Input: part model. Units: mm. Frame: model coordinates. A direction names the side the tool comes from. Coordinates: 2 decimals unless noted, no trailing zeros. Loops run counter-clockwise (first coordinate to the right, second up) from the corner with the lowest first, then second, coordinate; pieces in that order, holes last. Notation, with made-up numbers: M -8,-15.5 L 29,-15.5 A9 cw 29,-2.5 Z; hole C 21.25,-36.5 d11. An arc over 180 degrees is marked long. Use a Markdown table: item, result. Add a question column.
1. Section C-C on x = -12.5. Output: boundary loops of the cut face in (y, z), then the cut area to 3 significant figures.
2. Set-up query: faces 5 (the flat face through (0, -37, 1)), 6 (the cylindrical face through (-45.6, 35.5, 5)), 7 (the cylindrical face through (37.042, -47.174, 3.451)). Return all of +Z, -Z, +X, -X, +Y, -Y with unobstructed straight access to the full face (end or side cutting, diameter ignored); none if empty.
3. Line query: L1, parallel to Y at x = -10, z = 2; L2, parallel to X at y = -26.5, z = 5; L3, parallel to Y at x = 9, z = 6.5. Output: solid intervals per line, ascending. Write a range as [from, to].
4. Section B-B on z = 5.75. Output: boundary loops of the cut face in (x, y), then the cut area to 3 significant figures.
5. Section D-D on x = 19.5. Output: boundary loops of the cut face in (y, z).
6. Section A-A on y = -4. Output: boundary loops of the cut face in (x, z).
7. Pin query (flat end, axial travel): pin 1 (6 mm diameter, centred on x = 27, y = -1, fed in from +Z). Return the tip coordinate at first contact, or that it passes through.
8. Draft query along Y for faces 1 (the cylindrical face through (-41.951, 31.975, 1.521)), 2 (the cylindrical face through (-42.76, 21.16, 1.48)), 3 (the flat face through (14, -4, 0)), 4 (the cylindrical face through (-47.029, -47.096, 3.451)). Return one class per face: +Y half, -Y half, draft (parallel to the pull), parting line (faces both ways), or undercut.
```python
from build123d import *

# Parameters (mm, degrees)
F1_DEPTH = 3
F2_R     = 5
F3_R     = 5
F5_DEPTH = 4


with BuildPart() as f1:
    # F0 (on Top) → F1 (new body)
    with BuildSketch(Plane.XY):
        with BuildLine():
            Line((33.545249, 38.400311), (-43.454751, 38.400311))
            ThreePointArc((-43.454751, 38.400311), (-46.990285, 36.935845), (-48.454751, 33.400311))
            Line((-48.454751, 33.400311), (-48.454751, -43.599689))
            ThreePointArc((-48.454751, -43.599689), (-46.990285, -47.135222), (-43.454751, -48.599689))
            Line((-43.454751, -48.599689), (33.545249, -48.599689))
            ThreePointArc((33.545249, -48.599689), (37.080783, -47.135222), (38.545249, -43.599689))
            Line((38.545249, -43.599689), (38.545249, 33.400311))
            ThreePointArc((38.545249, 33.400311), (37.080783, 36.935845), (33.545249, 38.400311))
        make_face()
        with BuildLine():
            Line((-43.454751, 23.699071), (-43.454751, 33.400311))
            Line((-43.454751, 33.400311), (-2.236148, 33.400311))
            Line((-2.236148, 33.400311), (0, 33.400311))
            Line((0, 33.400311), (7.406416, 33.400311))
            ThreePointArc((7.406416, 33.400311), (8.481207, 33.201173), (9.41331, 32.630194))
            Line((9.41331, 32.630194), (11.244695, 30.981947))
            ThreePointArc((11.244695, 30.981947), (11.978301, 29.972581), (12.237801, 28.752065))
            Line((12.237801, 28.752065), (12.237801, 20.519217))
            ThreePointArc((12.237801, 20.519217), (11.877237, 19.093252), (10.882217, 18.010054))
            Line((10.882217, 18.010054), (9.100236, 16.842208))
            ThreePointArc((9.100236, 16.842208), (8.105216, 15.759011), (7.744652, 14.333046))
            Line((7.744652, 14.333046), (7.744652, -22.499491))
            ThreePointArc((7.744652, -22.499491), (7.265583, -24.635184), (5.920179, -26.361618))
            Line((5.920179, -26.361618), (1.824473, -29.729199))
            ThreePointArc((1.824473, -29.729199), (0.479069, -31.455634), (0, -33.591326))
            Line((0, -33.591326), (0, -40.599689))
            ThreePointArc((0, -40.599689), (-0.87868, -42.721009), (-3, -43.599689))
            Line((-3, -43.599689), (-43.454751, -43.599689))
            Line((-43.454751, -43.599689), (-43.454751, -32.622973))
            ThreePointArc((-43.454751, -32.622973), (-42.975682, -30.487281), (-41.630278, -28.760846))
            Line((-41.630278, -28.760846), (-34.385276, -22.803844))
            ThreePointArc((-34.385276, -22.803844), (-33.039872, -21.077409), (-32.560803, -18.941716))
            Line((-32.560803, -18.941716), (-32.560803, 11.657347))
            ThreePointArc((-32.560803, 11.657347), (-33.234097, 14.163262), (-35.072648, 15.994291))
            Line((-35.072648, 15.994291), (-40.942907, 19.362127))
            ThreePointArc((-40.942907, 19.362127), (-42.781458, 21.193155), (-43.454751, 23.699071))
        make_face(mode=Mode.SUBTRACT)
    extrude(amount=F1_DEPTH)

    # F2
    f2_edges = [f1.edges().sort_by_distance(p)[0] for p in [
        (-43.454751, 33.400311, 1.5),
    ]]
    fillet(f2_edges, radius=F2_R)

    # F3
    f3_edges = [f1.edges().sort_by_distance(p)[0] for p in [
        (-43.454751, -43.599689, 1.5),
    ]]
    fillet(f3_edges, radius=F3_R)

    # F4 (on face) → F5 (join)
    with BuildSketch(Plane.XY.offset(3)):
        with BuildLine():
            Line((33.545249, 38.400311), (-43.454751, 38.400311))
            ThreePointArc((-43.454751, 38.400311), (-46.990285, 36.935845), (-48.454751, 33.400311))
            Line((-48.454751, 33.400311), (-48.454751, -43.599689))
            ThreePointArc((-48.454751, -43.599689), (-46.990285, -47.135222), (-43.454751, -48.599689))
            Line((-43.454751, -48.599689), (33.545249, -48.599689))
            ThreePointArc((33.545249, -48.599689), (37.080783, -47.135222), (38.545249, -43.599689))
            Line((38.545249, -43.599689), (38.545249, 33.400311))
            ThreePointArc((38.545249, 33.400311), (37.080783, 36.935845), (33.545249, 38.400311))
        make_face()
        with BuildLine():
            ThreePointArc((-46.454751, 33.400311), (-45.576071, 35.521631), (-43.454751, 36.400311))
            Line((-43.454751, 36.400311), (33.545249, 36.400311))
            ThreePointArc((33.545249, 36.400311), (35.666568, 35.521631), (36.545248, 33.400311))
            Line((36.545248, 33.400311), (36.545248, -43.599689))
            ThreePointArc((36.545248, -43.599689), (35.666568, -45.721008), (33.545249, -46.599688))
            Line((33.545249, -46.599688), (-43.454751, -46.599688))
            ThreePointArc((-43.454751, -46.599688), (-45.576071, -45.721008), (-46.454751, -43.599689))
            Line((-46.454751, -43.599689), (-46.454751, 33.400311))
        make_face(mode=Mode.SUBTRACT)
    extrude(amount=F5_DEPTH)


solid = f1.part
```
Answers below:
| question | item | result |
|---|---|---|
| 1 | outline | M -48.6,0 L -43.6,0 L -43.6,3 L -46.6,3 L -46.6,7 L -48.6,7 Z; M 33.4,0 L 38.4,0 L 38.4,7 L 36.4,7 L 36.4,3 L 33.4,3 Z |
| 1 | area | 46.0 mm² |
| 2 | face 5 | +Z, -Z |
| 2 | face 6 | +Z |
| 2 | face 7 | +Z, -Z, +X, -Y |
| 3 | L1 | y = [-48.6, -43.6], [33.4, 38.4] |
| 3 | L2 | x = [-48.45, -46.45], [36.55, 38.55] |
| 3 | L3 | y = [-48.6, -46.6], [36.4, 38.4] |
| 4 | outline | M -48.45,-43.6 A5 ccw -43.45,-48.6 L 33.55,-48.6 A5 ccw 38.55,-43.6 L 38.55,33.4 A5 ccw 33.55,38.4 L -43.45,38.4 A5 ccw -48.45,33.4 Z; hole M -46.45,-43.6 A3 ccw -43.45,-46.6 L 33.55,-46.6 A3 ccw 36.55,-43.6 L 36.55,33.4 A3 ccw 33.55,36.4 L -43.45,36.4 A3 ccw -46.45,33.4 Z |
| 4 | area | 666 mm² |
| 5 | outline | M -48.6,0 L 38.4,0 L 38.4,7 L 36.4,7 L 36.4,3 L -46.6,3 L -46.6,7 L -48.6,7 Z |
| 6 | outline | M -48.45,0 L -32.56,0 L -32.56,3 L -46.45,3 L -46.45,7 L -48.45,7 Z; M 7.74,0 L 38.55,0 L 38.55,7 L 36.55,7 L 36.55,3 L 7.74,3 Z |
| 7 | pin 1 | stops at z = 3 |
| 8 | face 1 | undercut |
| 8 | face 2 | undercut |
| 8 | face 3 | draft |
| 8 | face 4 | -Y half |
